Part model, mm, in its own coordinate system. Face numbers are marked on the shaded views. Round coordinates to 2 decimals unless told otherwise and drop trailing zeros. Order: outer loops, then holes, each group sorted by start corner. A loop starts at its lowest first (then second) coordinate and runs counter-clockwise, first axis right, second up. Notation, with made-up numbers: (7.25, -17) - (51.25, -17) arc R22 cw to (51.25, -5) - close; hole circle Ø2 at (44, 6.5). An arc over 180 degrees is marked (long way). Return JSON: item names as keys, results as strings. Group by question number.
Item 1: Saw through at B-B on z = 4.5. List the corners of the cut face in (x, y).
Item 2: Drop a flat-ended pin along its axis: pin 1 (3.5 mm diameter, centred on x = 0, y = 0, fed in from +Z). Give the stop position or say it passes through.
Item 3: Probe probe 1 along Z at (x, y) = (4.25, 0); probe 2 along Z at (x, y) = (-3.5, -1). List the from-to ranges inside material, lowest first.
Item 4: Saw through at C-C on z = -2. List the corners of the cut face in (x, y), and give its area (3 significant figures).
Item 5: Saw through at D-D on y = -2.5. List the corners of the cut face in (x, z).
Item 6: Two-plate mould, pull along Z, no slides. Class the marked faces 1, 2 and 3: released by +Z, released by -Z, zero draft, split by the parting line, or undercut.
Item 7: Saw through at A-A on y = 0. List the corners of the cut face in (x, z), and give its area (3 significant figures).
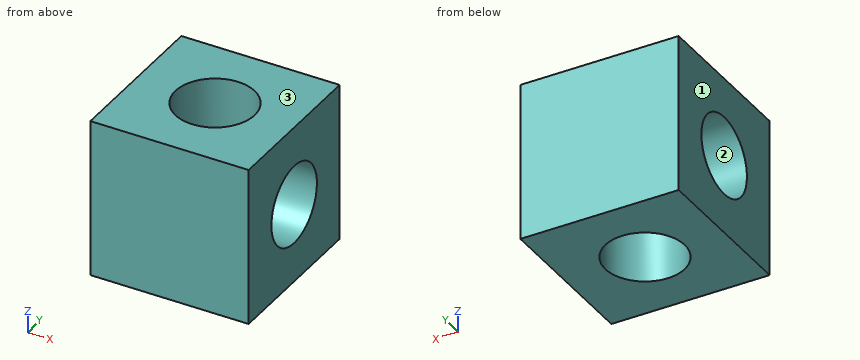
```python
from build123d import *

# Parameters (mm, degrees)
SKETCH1_W          = 19.05
SKETCH1_H          = 19.05
SKETCH1_R          = 4.7625
BASE_EXTRUDE_DEPTH = 9.525
SKETCH3_R          = 4.7625
CUT_EXTRUDE1_DEPTH = 24.3313898
SCALE1_SCALE       = 0.65


with BuildPart() as part:
    # Sketch1 → Base-Extrude (new, symmetric)
    with BuildSketch(Plane.XY):
        Rectangle(SKETCH1_W, SKETCH1_H)
        with Locations(Location((0, 0, 0), (0, 0, 180))):
            Circle(SKETCH1_R, mode=Mode.SUBTRACT)
    extrude(amount=BASE_EXTRUDE_DEPTH, both=True)

    # Sketch3 → Cut-Extrude1 (cut, through all)
    with BuildSketch(Plane(origin=(9.525, 0, 0), x_dir=(0, 0, -1), z_dir=(1, 0, 0))):
        Circle(SKETCH3_R)
    extrude(amount=-CUT_EXTRUDE1_DEPTH, mode=Mode.SUBTRACT)


with BuildPart() as part_1:
    # Scale1: scaled about (0, 0, 0)
    add(part.part.scale(SCALE1_SCALE))


solid = part_1.part
```
Filled in:
{
 "1": {"outline": "(-6.19, -6.19) - (6.19, -6.19) - (6.19, 6.19) - (-6.19, 6.19) - close; hole circle Ø6.19 at (0, 0)"},
 "2": {"pin 1": "passes through"},
 "3": {"probe 1": "z = -6.19 to -3.1, 3.1 to 6.19", "probe 2": "z = -6.19 to -2.93, 2.93 to 6.19"},
 "4": {"outline": "(-6.19, -6.19) - (6.19, -6.19) - (6.19, -2.36) - (2, -2.36) arc R3.1 cw to (-2, -2.36) - (-6.19, -2.36) - close; (-6.19, 2.36) - (-2, 2.36) arc R3.1 cw to (2, 2.36) - (6.19, 2.36) - (6.19, 6.19) - (-6.19, 6.19) - close", "area": "90.8 mm^2"},
 "5": {"outline": "(-6.19, -6.19) - (-1.83, -6.19) - (-1.83, -1.83) - (-6.19, -1.83) - close; (-6.19, 1.83) - (-1.83, 1.83) - (-1.83, 6.19) - (-6.19, 6.19) - close; (1.83, -6.19) - (6.19, -6.19) - (6.19, -1.83) - (1.83, -1.83) - close; (1.83, 1.83) - (6.19, 1.83) - (6.19, 6.19) - (1.83, 6.19) - close"},
 "6": {"face 1": "zero draft", "face 2": "undercut", "face 3": "released by +Z"},
 "7": {"outline": "(-6.19, -6.19) - (-3.1, -6.19) - (-3.1, -3.1) - (-6.19, -3.1) - close; (-6.19, 3.1) - (-3.1, 3.1) - (-3.1, 6.19) - (-6.19, 6.19) - close; (3.1, -6.19) - (6.19, -6.19) - (6.19, -3.1) - (3.1, -3.1) - close; (3.1, 3.1) - (6.19, 3.1) - (6.19, 6.19) - (3.1, 6.19) - close", "area": "38.3 mm^2"}
}
